from build123d import *

# Parameters (mm, degrees)
SKETCH_1_W      = 86
SKETCH_1_H      = 62
EXTRUDE_1_DEPTH = 3
SKETCH_2_W      = 74
SKETCH_2_H      = 52
EXTRUDE_2_DEPTH = 1
FILLET_1_R      = 5
FILLET_2_R      = 2


with BuildPart() as part:
    # 草图1 → 凸台-拉伸1 (new body)
    with BuildSketch(Plane(origin=(0, 0, 0), x_dir=(1, 0, 0), z_dir=(0, 1, 0))):
        Rectangle(SKETCH_1_W, SKETCH_1_H)
    extrude(amount=EXTRUDE_1_DEPTH)

    # 草图2 → 凸台-拉伸2 (add)
    with BuildSketch(Plane(origin=(0, 3, 0), x_dir=(1, 0, 0), z_dir=(0, 1, 0))):
        Rectangle(SKETCH_2_W, SKETCH_2_H)
    extrude(amount=EXTRUDE_2_DEPTH)

    # 圆角1
    fillet_1_edges = [part.edges().sort_by_distance(p)[0] for p in [
        (-43, 1.5, -31),
        (43, 1.5, -31),
        (43, 1.5, 31),
        (-43, 1.5, 31),
    ]]
    fillet(fillet_1_edges, radius=FILLET_1_R)

    # 圆角2
    fillet_2_edges = [part.edges().sort_by_distance(p)[0] for p in [
        (-37, 3.5, -26),
        (-37, 3.5, 26),
        (37, 3.5, 26),
        (37, 3.5, -26),
    ]]
    fillet(fillet_2_edges, radius=FILLET_2_R)


solid = part.part
Model file for the job. Use its own axes, mm. A direction names the side the tool comes from. Coordinates: 2 decimals unless noted, no trailing zeros. Order: outer loops, then holes, each group sorted by start corner. A loop starts at its lowest first (then second) coordinate and runs counter-clockwise, first axis right, second up. Notation, with made-up numbers: M -15.75,-3.5 L 38.25,-3.5 A11 ccw 38.25,16.5 Z; hole C 14,-33.5 d7. An arc over 180 degrees is marked long. Return JSON: item names as keys, results as strings.
1. Drill centre lines: probe 1 along Z at (x, y) = (24.5, 3.35); probe 2 along X at (y, z) = (3.35, -19.5); probe 3 along Z at (x, y) = (-39, 0.5). Where is each one in solid material? Low to high.
Ans:
{"probe 1": "-26 to 26", "probe 2": "-37 to 37", "probe 3": "-30.9 to 30.9"}
2. Saw through at B-B (x = 25). Give the cut face in (y, z), and give its area (3 significant figures).
Ans:
{"outline": "M 0,-31 L 3,-31 L 3,-26 L 4,-26 L 4,26 L 3,26 L 3,31 L 0,31 Z", "area": "238 mm^2"}
3. Tool access for faces 1 (the face through (36.43, 3.51, -25.4)), 2 (the face through (-1, 3, 27)), 3 (the face through (36.4, 3.51, 25.43)), 4 (the face through (-36.4, 3.51, 25.43)), 5 (the face through (-36.4, 3.51, -25.43)): list every direction of +Z, -Z, +X, -X, +Y, -Y with a clear straight run to the whole face (end or side of a thin tool).
Ans:
{"face 1": "-Z, +X, +Y", "face 2": "+Y", "face 3": "+Z, +X, +Y", "face 4": "+Z, -X, +Y", "face 5": "-Z, -X, +Y"}
4. Saw through at A-A (z = 3.5). Give the cut face in (x, y), and give its area (3 significant figures).
Ans:
{"outline": "M -43,0 L 43,0 L 43,3 L 37,3 L 37,4 L -37,4 L -37,3 L -43,3 Z", "area": "332 mm^2"}
5. Flat gauge pins, fed straight in: pin 1 (0.8 mm diameter, centred on y = 3.5, z = 10, fed in from -X); pin 2 (1.1 mm diameter, centred on x = -9, y = 3.5, fed in from -Z). Where does each tip first touch, or does it go through?
Ans:
{"pin 1": "x = -37", "pin 2": "z = -31"}
